Part model, mm, in its own coordinate system. Face numbers are marked on the shaded views. Round coordinates to 2 decimals unless told otherwise and drop trailing zeros. Loops run counter-clockwise (first coordinate to the right, second up) from the corner with the lowest first, then second, coordinate; pieces in that order, holes last.
1) Mould opens along Z. For the marked faces 1 and 2 say: +Z half, -Z half, draft (parallel to the pull), parting line (faces both ways), or undercut.
2) Probe line 1 (Y direction, x = 0, z = -5.3); line 2 (X direction, y = 111, z = 0). List the from-to ranges inside material, lowest first.
3) Band-saw the part on C-C, the plane z = 0. Write the cut outline in (x, y).
4) Band-saw the part on D-D, the plane y = 27.5. Write the cut outline in (x, z), then the cut area to 3 significant figures.
5) Drop flat-ended pins along their axis: P1, Ø4.5, axis at x = 0, y = 5, coming from the -Z side; P2, Ø0.9, axis at y = 101, z = -5, coming from the -X side; P3, Ø1.2, axis at y = 88, z = 4.5, coming from the +X side; P4, Ø1.5, axis at y = 104, z = 3, coming from the +X side. Give the stop position or say it passes through.
6) Band-saw the part on A-A, the plane y = 145. Write the cut outline in (x, z), then the cut area to 3 significant figures.
7) Band-saw the part on B-B, the plane x = 0. State how many separate pieces and enclosed holes the cut face has, then the cut area to 3 significant figures.
from build123d import *

# Parameters (mm, degrees)
SZKIC1_R                        = 6
SZKIC1_R_2                      = 5
DODANIE_WYCI_GNI_CIE1_DEPTH     = 150
SZKIC3_R                        = 2.5
WYTNIJ_WYCI_GNI_CIE2_DEPTH      = 7
WYTNIJ_WYCI_GNI_CIE2_DEPTH_BACK = 7


with BuildPart() as part:
    # Szkic1 → Dodanie-wyciągnięcie1 (new body)
    with BuildSketch(Plane(origin=(0, 0, 0), x_dir=(1, 0, 0), z_dir=(0, 1, 0))):
        Circle(SZKIC1_R)
        Circle(SZKIC1_R_2, mode=Mode.SUBTRACT)
    extrude(amount=DODANIE_WYCI_GNI_CIE1_DEPTH)

    # Szkic3 → Wytnij-wyciągnięcie2 (cut, two sides)
    with BuildSketch(Plane.XY) as wytnij_wyci_gni_cie2_sk:
        with Locations((0, 145)):
            Circle(SZKIC3_R)
        with Locations((0, 5)):
            Circle(SZKIC3_R)
        with BuildLine():
            Line((-2.5, 79.5), (-2.5, 109.5))
            ThreePointArc((-2.5, 109.5), (0, 112), (2.5, 109.5))
            Line((2.5, 109.5), (2.5, 79.5))
            ThreePointArc((2.5, 79.5), (0, 77), (-2.5, 79.5))
        make_face()
    extrude(amount=WYTNIJ_WYCI_GNI_CIE2_DEPTH, mode=Mode.SUBTRACT)
    extrude(wytnij_wyci_gni_cie2_sk.sketch, amount=-WYTNIJ_WYCI_GNI_CIE2_DEPTH_BACK, mode=Mode.SUBTRACT)


solid = part.part
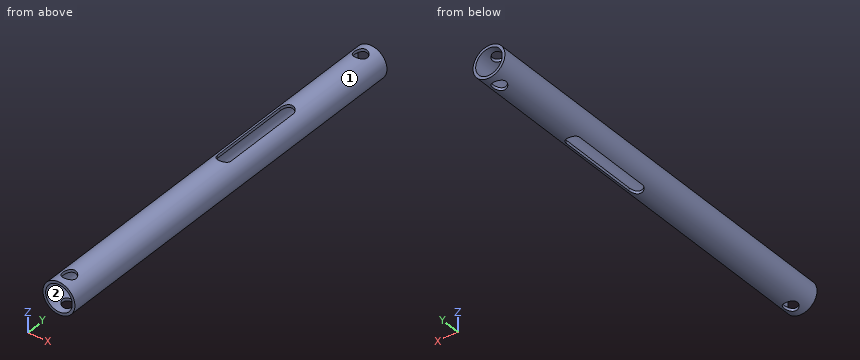
Reported:
1. face 1: parting line
1. face 2: undercut
2. line 1: y = 0 to 2.5, 7.5 to 77, 112 to 142.5, 147.5 to 150
2. line 2: x = -6 to -5, 5 to 6
3. outline: (-6, 0) - (-5, 0) - (-5, 150) - (-6, 150) - close; (5, 0) - (6, 0) - (6, 150) - (5, 150) - close
4. outline: circle Ø12 at (0, 0); hole circle Ø10 at (0, 0)
4. area: 34.6 mm2
5. P1: passes through
5. P2: stops at x = -3.91
5. P3: stops at x = 4.56
5. P4: stops at x = 5.56
6. outline: (-2.5, -5.45) - (-2.5, -4.33) arc R5 cw to (-2.5, 4.33) - (-2.5, 5.45) arc R6 ccw to start; (2.5, -5.45) arc R6 ccw to (2.5, 5.45) - (2.5, 4.33) arc R5 cw to (2.5, -4.33) - close
6. area: 24.2 mm2
7. separate pieces: 8
7. enclosed holes: 0
7. area: 210 mm2
